Read the model definition and answer for the solid it produces. Units are mm, in the model's axes. Coordinates: 2 decimals unless noted, no trailing zeros. Loops run counter-clockwise (first coordinate to the right, second up) from the corner with the lowest first, then second, coordinate; pieces in that order, holes last. Notation, with made-up numbers: M 39.25,-18.5 L 65.25,-18.5 A15 cw 65.25,-14.5 Z; hole C -16,-13 d9. An arc over 180 degrees is marked long. One line per item, written item: value. Start each with the question number.
1. Determine the mould class of faces 1 (the face through (1, 2, -30.48)), 2 (the face through (1, 2, 2.54)), 3 (the face through (0.6, 0.54, -14.2)), 4 (the face through (0, 2, -14)) for opening direction Z: +Z half, -Z half, draft (parallel to the pull), parting line (faces both ways), or undercut.
2. Flat-ended cylindrical pins translate along their axes: pin 1 (0.7 mm diameter, centred on y = 7, z = -26.5, fed in from -X); pin 2 (1 mm diameter, centred on x = 1.5, z = -25.5, fed in from -Y); pin 3 (0.5 mm diameter, centred on x = 1, y = 6.5, fed in from +Z). Find the tip coordinate at first contact, or state that the pin passes through.
3. The part is cut by section A-A (y = 6). State how many separate pieces and enclosed holes the cut face has, then the cut area to 3 significant figures.
4. The part is cut by section B-B (z = -17.5). Write down the section's boundary in (x, y).
5. The part is cut by section C-C (x = 0.6). Write down the section's boundary in (y, z).
6. Consider probe 1 along X at (y, z) = (7.75, -1.5); probe 2 along Y at (x, z) = (1.7, -22); probe 3 along Y at (x, z) = (2.3, -11.5). Determine where each line is inside the solid, lowest interval first.
```python
from build123d import *

# Parameters (mm, degrees)
EXTRUDE_1_DEPTH            = 2.54
EXTRUDE_START              = -5.5
SKETCH_2_W                 = 0.64
SKETCH_2_H                 = 0.64
EXTRUDE_2_DEPTH            = 11.5
PATTERN_LINEAR_27_COUNT    = 13
PATTERN_LINEAR_27_PITCH    = 2.54
CROQUIS1_W                 = 6.114803871
CROQUIS1_H                 = 33.02
CORTAR_EXTRUIR1_DEPTH      = 9.54
CORTAR_EXTRUIR1_DEPTH_BACK = 3.96


with BuildPart() as part:
    # Эскиз1 → Бобышка-Вытянуть1 (new body)
    with BuildSketch(Plane.XY):
        Polygon((-2.54, 0), (-2.54, 2.54), (2.54, 2.54), (2.54, 0), (2.04, 0), (2.04, 0.54), (-2.04, 0.54), (-2.04, 0), align=None)
    extrude_1 = extrude(amount=EXTRUDE_1_DEPTH)

    # Эскиз2 → Бобышка-Вытянуть2 (add)
    with BuildSketch(Plane(origin=(0, 2.54, 0), x_dir=(1, 0, 0), z_dir=(0, 1, 0)).offset(EXTRUDE_START)):
        with Locations((-1.27, -1.27)):
            Rectangle(SKETCH_2_W, SKETCH_2_H)
        with Locations((1.27, -1.27)):
            Rectangle(SKETCH_2_W, SKETCH_2_H)
    extrude_2 = extrude(amount=EXTRUDE_2_DEPTH)

    # Линейный массив27: Бобышка-Вытянуть1, Бобышка-Вытянуть2 ×13
    with Locations(*[(0, 0, -i * PATTERN_LINEAR_27_PITCH) for i in range(1, PATTERN_LINEAR_27_COUNT)]):
        add(extrude_1)
        add(extrude_2)

    # Croquis1 → Cortar-Extruir1 (cut, two sides)
    with BuildSketch(Plane(origin=(0, 0, 0), x_dir=(1, 0, 0), z_dir=(0, 1, 0))) as cortar_extruir1_sk:
        with Locations((-3.057401936, 13.97)):
            Rectangle(CROQUIS1_W, CROQUIS1_H)
    extrude(amount=CORTAR_EXTRUIR1_DEPTH, mode=Mode.SUBTRACT)
    extrude(cortar_extruir1_sk.sketch, amount=-CORTAR_EXTRUIR1_DEPTH_BACK, mode=Mode.SUBTRACT)


solid = part.part
```
Answer block:
1. face 1: -Z half
1. face 2: +Z half
1. face 3: undercut
1. face 4: draft
2. pin 1: stops at x = 0.95
2. pin 2: stops at y = 0.54
2. pin 3: stops at z = 1.59
3. separate pieces: 13
3. enclosed holes: 0
3. area: 5.32 mm2
4. outline: M 0,0.54 L 2.04,0.54 L 2.04,0 L 2.54,0 L 2.54,2.54 L 0,2.54 Z
5. outline: M 0.54,-30.48 L 2.54,-30.48 L 2.54,2.54 L 0.54,2.54 Z
6. probe 1: x = 0.95 to 1.59
6. probe 2: y = 0.54 to 2.54
6. probe 3: y = 0 to 2.54
